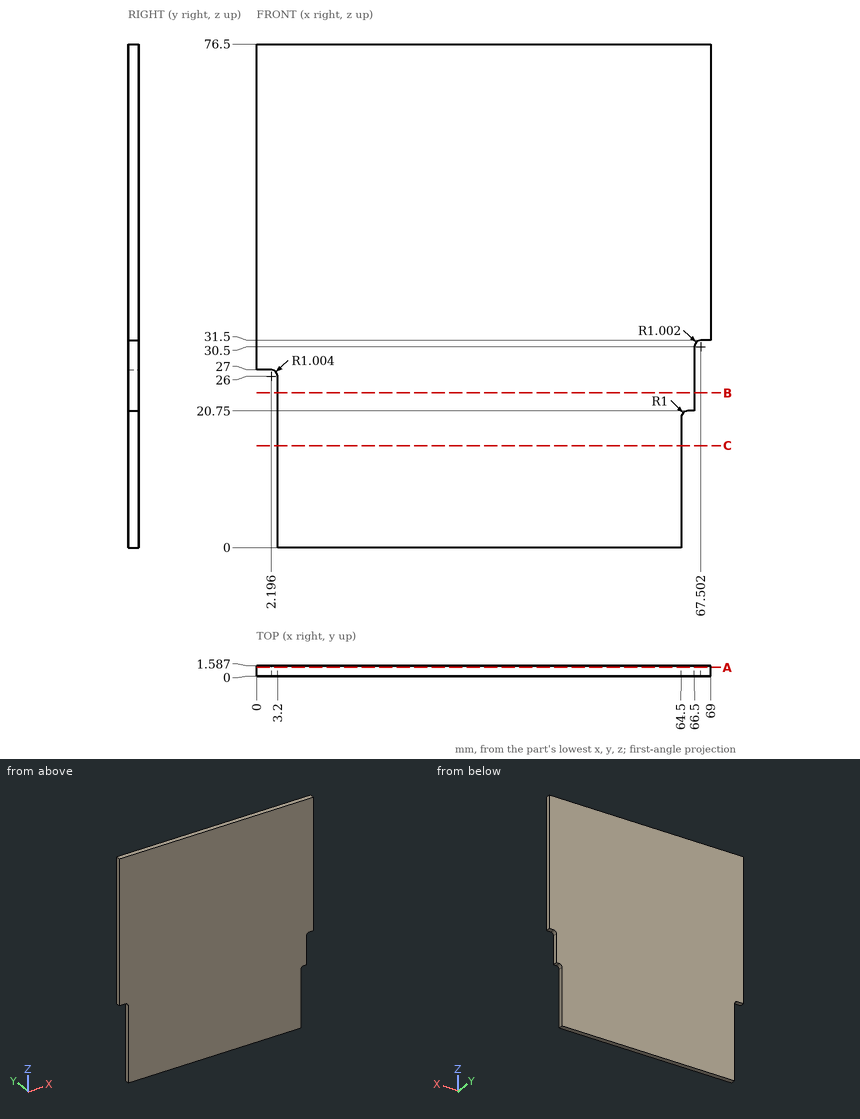
The drawing under review shows one solid part. Ordinate dimensions are in mm from its lowest x, y, z. Give positions to 0.01 mm unless a question says otherwise; leave off trailing zeros. Write each loop counter-clockwise with the first axis right and the second up, starting at its lowest first coordinate (ties: lowest second). Pieces come first, ordered by that corner, then holes. Notation, with made-up numbers: (4, 68) - (25, 68) arc R20 cw to (25, 87) - close; hole circle Ø8 at (75.5, 14.25). An arc over 180 degrees is marked (long way). Answer in a Markdown table with one row per item. Add a question column.
1. Insertion check: P1, Ø4, axis at x = 58, z = 10.5, coming from the -Y side; P2, Ø0.5, axis at y = 0.5, z = 12, coming from the -X side; P3, Ø0.5, axis at x = 1, y = 0.5, coming from the -Z side; P4, Ø0.5, axis at y = 0.5, z = 14.5, coming from the +X side. Each pin has a flat end and moves straight along its axis. Give the tip position at first contact, or say it passes through.
2. We need section B-B on z = 23.5. Write out the cut boundary in (x, y).
3. Wall thickness on line 1 along X through (y, z) = (1.1, 30.5); line 2 along X through (y, z) = (1.2, 23): over which ranges is each line inside the solid? List them lowest first. Write a range as [from, to].
4. We need section C-C on z = 15.5. Write out the cut boundary in (x, y).
5. We need section A-A on y = 1.3. Write out the cut boundary in (x, z).
Ans:
| question | item | result |
|---|---|---|
| 1 | P1 | stops at y = 0 |
| 1 | P2 | stops at x = 3.2 |
| 1 | P3 | stops at z = 27 |
| 1 | P4 | stops at x = 64.5 |
| 2 | outline | (3.2, 0) - (66.5, 0) - (66.5, 1.59) - (3.2, 1.59) - close |
| 3 | line 1 | x = [0, 66.5] |
| 3 | line 2 | x = [3.2, 66.5] |
| 4 | outline | (3.2, 0) - (64.5, 0) - (64.5, 1.59) - (3.2, 1.59) - close |
| 5 | outline | (0, 27) - (2.28, 27) arc R1 cw to (3.2, 26) - (3.2, 0) - (64.5, 0) - (64.5, 19.75) arc R1 cw to (65.5, 20.75) - (66.5, 20.75) - (66.5, 30.5) arc R1 cw to (67.44, 31.5) - (69, 31.5) - (69, 76.5) - (0, 76.5) - close |
